from build123d import *

# Parameters (mm, degrees)
BOSS_EXTRUDE1_DEPTH = 127
SKETCH4_R           = 1.651
CUT_EXTRUDE1_DEPTH  = 130.554006596
SKETCH5_R           = 1.651
CUT_EXTRUDE2_DEPTH  = 130.554006596
SKETCH4_5_R         = 1.651
SKETCH4_5_R_2       = 6.35
SKETCH4_5_R_3       = 6.323800798
SKETCH4_5_R_4       = 6.460876205
CUT_EXTRUDE3_DEPTH  = 130.554006596


with BuildPart() as part:
    # Sketch2 → Boss-Extrude1 (new, symmetric)
    with BuildSketch(Plane.XY):
        with BuildLine():
            Line((-12.7, -12.7), (12.7, -12.7))
            Line((12.7, -12.7), (12.7, 12.7))
            Line((12.7, 12.7), (11.1125, 12.7))
            ThreePointArc((11.1125, 12.7), (9.989967985, 12.235032015), (9.525, 11.1125))
            Line((9.525, 11.1125), (9.525, -6.35))
            ThreePointArc((9.525, -6.35), (8.59506403, -8.59506403), (6.35, -9.525))
            Line((6.35, -9.525), (-11.1125, -9.525))
            ThreePointArc((-11.1125, -9.525), (-12.235032015, -9.989967985), (-12.7, -11.1125))
            Line((-12.7, -11.1125), (-12.7, -12.7))
        make_face()
    extrude(amount=BOSS_EXTRUDE1_DEPTH, both=True)

    # Sketch4 → Cut-Extrude1 (cut, through all)
    with BuildSketch(Plane(origin=(0, -9.525, 0), x_dir=(1, 0, 0), z_dir=(0, 1, 0))):
        with Locations(Location((-5.55625, 101.6, 0), (0, 0, 180))):
            Circle(SKETCH4_R)
        with Locations(Location((0.79375, 88.907891862, 0), (0, 0, 180))):
            Circle(SKETCH4_R)
        with Locations((0.79375, -88.907891862)):
            Circle(SKETCH4_R)
        with Locations((-5.55625, -101.6)):
            Circle(SKETCH4_R)
    extrude(amount=-CUT_EXTRUDE1_DEPTH, mode=Mode.SUBTRACT)

    # Sketch5 → Cut-Extrude2 (cut, through all)
    with BuildSketch(Plane.ZY.offset(-9.525)):
        with Locations(Location((-88.9, 5.55625, 0), (0, 0, 270))):
            Circle(SKETCH5_R)
        with Locations(Location((-101.6, -0.79375, 0), (0, 0, 270))):
            Circle(SKETCH5_R)
        with Locations(Location((88.9, 5.55625, 0), (0, 0, 90))):
            Circle(SKETCH5_R)
        with Locations(Location((101.6, -0.79375, 0), (0, 0, 90))):
            Circle(SKETCH5_R)
    extrude(amount=-CUT_EXTRUDE2_DEPTH, mode=Mode.SUBTRACT)

    # Sketch4_5 → Cut-Extrude3 (cut, through all)
    with BuildSketch(Plane(origin=(0, -9.525, 0), x_dir=(1, 0, 0), z_dir=(0, 1, 0))):
        with Locations(Location((-5.55625, 101.6, 0), (0, 0, 180))):
            Circle(SKETCH4_5_R)
        with Locations(Location((0.79375, 88.907891862, 0), (0, 0, 180))):
            Circle(SKETCH4_5_R)
        with Locations((0.79375, -88.907891862)):
            Circle(SKETCH4_5_R)
        with Locations((-5.55625, -101.6)):
            Circle(SKETCH4_5_R)
        with Locations(Location((-2.38125, 77.702134885, 0), (0, 0, 180))):
            Circle(SKETCH4_5_R_2)
        with Locations(Location((-2.222550137, 58.755442455, 0), (0, 0, 180))):
            Circle(SKETCH4_5_R_3)
        with Locations(Location((-2.061352022, 38.605678066, 0), (0, 0, 180))):
            Circle(SKETCH4_5_R_3)
        with Locations(Location((-2.383748252, 20.551489173, 0), (0, 0, 180))):
            Circle(SKETCH4_5_R_3)
        with Locations(Location((-2.38125, 0, 0), (0, 0, 180))):
            Circle(SKETCH4_5_R_4)
        with Locations((-2.061352022, -38.605678066)):
            Circle(SKETCH4_5_R_3)
        with Locations((-2.383748252, -20.551489173)):
            Circle(SKETCH4_5_R_3)
        with Locations((-2.222550137, -58.755442455)):
            Circle(SKETCH4_5_R_3)
        with Locations((-2.38125, -77.702134885)):
            Circle(SKETCH4_5_R_2)
    extrude(amount=-CUT_EXTRUDE3_DEPTH, mode=Mode.SUBTRACT)


solid = part.part
Could you check a few things on this model? Use its own coordinates, in mm. A direction names the side the tool comes from. Coordinates: 2 decimals unless noted, no trailing zeros.
1. I need wall thicknesses on L1, parallel to Z at x = 10.25, y = 7; L2, parallel to Y at x = 11.7, z = -101.6; L3, parallel to X at y = -10.75, z = 101.6. Which ranges of each line are inside material? Lowest first, please.
2. We'd pull the mould along X, two halves only. Please class faces 1 (the face through (12.7, 0, 2)), 2 (the face through (-1.238, -11.09, -32.336)), 3 (the face through (5, -12.7, 2)), 4 (the face through (9.525, 3, 2)): released by +X, released by -X, zero draft, split by the parting line, or undercut.
3. For faces 5 (the face through (-10, -9.525, 2)), 6 (the face through (-5.363, -11.09, -5.732)), which set-ups out of +Z, -Z, +X, -X, +Y, -Y let a thin tool reach every point of the face, with its end or its side?
4. For P1, Ø14, axis at x = -4, z = -45.5, coming from the +Y side (3 decimals); P2, Ø14, axis at y = -1, z = 58.5, coming from the -X side; P3, Ø6, axis at y = -1, z = -47, coming from the -X side (3 decimals), each with a flat end and sliding along its axis, tell me the tip position at first contact or that it passes through.
Computed values:
1. L1: z = -127 to -89.7, -88.1 to 88.1, 89.7 to 127
1. L2: y = -12.7 to -2.44, 0.86 to 12.7
1. L3: x = -12.66 to -7.21, -3.91 to 12.7
2. face 1: released by +X
2. face 2: undercut
2. face 3: zero draft
2. face 4: released by -X
3. face 5: +Z, -Z, -X, +Y
3. face 6: +Y, -Y
4. P1: stops at y = -9.525
4. P2: stops at x = 9.06
4. P3: stops at x = 9.525
